Work out the finished part from the listing and answer in its coordinate system (mm). Face numbers are marked on the shaded views. Give positions to 0.01 mm unless a question says otherwise; leave off trailing zeros. Loops run counter-clockwise (first coordinate to the right, second up) from the corner with the lowest first, then second, coordinate; pieces in that order, holes last. Notation, with made-up numbers: (78, 76.5) - (132, 76.5) arc R23 ccw to (132, 94.5) - close; hole circle Ø6 at (89, -28.75). An arc over 180 degrees is marked (long way). One line per question, with ' | ' between items.
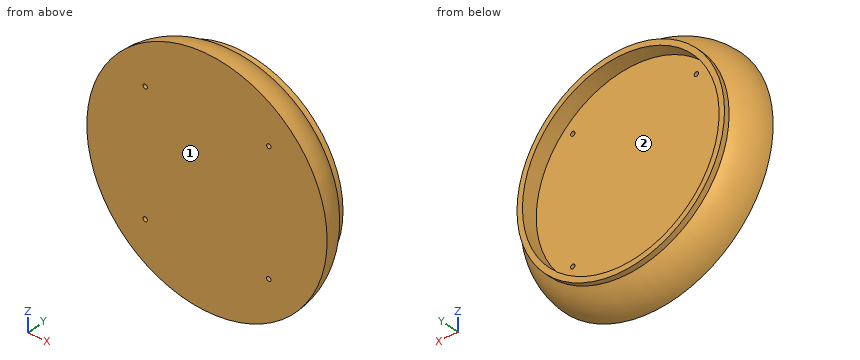
from build123d import *

# Parameters (mm, degrees)
SKETCH1_R          = 2
CUT_EXTRUDE1_DEPTH = 21


with BuildPart() as part:
    # Sketch2 → Revolve1 (revolve)
    with BuildSketch(Plane.XY):
        with BuildLine():
            Line((90, 0), (90, 15))
            Line((90, 15), (95, 15))
            Line((95, 15), (95, 10))
            ThreePointArc((95, 10), (106.041019662, -3.229490169), (110, -20))
            Line((110, -20), (0, -20))
            Line((0, -20), (0, 0))
            Line((0, 0), (90, 0))
        make_face()
    revolve(axis=Axis((0, 0, 0), (0, -1, 0)))

    # Sketch1 → Cut-Extrude1 (cut, through all)
    with BuildSketch(Plane(origin=(0, 0, 0), x_dir=(1, 0, 0), z_dir=(0, 1, 0))):
        with Locations((-56.568542495, 56.568542495)):
            Circle(SKETCH1_R)
        with Locations((-56.568542495, -56.568542495)):
            Circle(SKETCH1_R)
        with Locations((56.568542495, 56.568542495)):
            Circle(SKETCH1_R)
        with Locations((56.568542495, -56.568542495)):
            Circle(SKETCH1_R)
    extrude(amount=-CUT_EXTRUDE1_DEPTH, mode=Mode.SUBTRACT)


solid = part.part
1. Find section B-B on z = 0. Write down the section's boundary in (x, y), then the cut area to 3 significant figures.
Evaluation:
outline: (-110, -20) - (110, -20) arc R37.5 ccw to (95, 10) - (95, 15) - (90, 15) - (90, 0) - (-90, 0) - (-90, 15) - (-95, 15) - (-95, 10) arc R37.5 ccw to start | area: 4,580 mm2
2. Flat-ended cylindrical pins translate along their axes: pin 1 (4.5 mm diameter, centred on x = 56.57, z = 56.57, fed in from -Y); pin 2 (2 mm diameter, centred on y = -15.5, z = -26, fed in from -X); pin 3 (3 mm diameter, centred on x = 64, z = 37, fed in from +Y); pin 4 (4 mm diameter, centred on y = 10, z = -54.5, fed in from +X). Find the tip coordinate at first contact, or state that the pin passes through.
Evaluation:
pin 1: y = -20 | pin 2: x = -106.87 | pin 3: y = 0 | pin 4: x = 81.09
3. Find section C-C on y = -5. Write down the section's boundary in (x, z), then the cut area to 3 significant figures.
Evaluation:
outline: circle Ø213.74 at (0, 0); hole circle Ø4 at (-56.57, -56.57); hole circle Ø4 at (-56.57, 56.57); hole circle Ø4 at (56.57, -56.57); hole circle Ø4 at (56.57, 56.57) | area: 35,800 mm2
4. Consider L1, parallel to Z at x = -55, y = -5; L2, parallel to X at y = -15, z = -58; L3, parallel to Y at x = 10, z = 48.5. Determine where each line is inside the solid, lowest interval first.
Evaluation:
L1: -91.63 to -57.81, -55.33 to 55.33, 57.81 to 91.63 | L2: -93.07 to -57.97, -55.17 to 55.17, 57.97 to 93.07 | L3: -20 to 0
5. Find section A-A on x = 0. Write down the section's boundary in (y, z).
Evaluation:
outline: (-20, -110) arc R37.5 ccw to (10, -95) - (15, -95) - (15, -90) - (0, -90) - (0, 90) - (15, 90) - (15, 95) - (10, 95) arc R37.5 ccw to (-20, 110) - close
6. Determine the mould class of the marked faces 1 and 2 for opening direction Z: +Z half, -Z half, draft (parallel to the pull), parting line (faces both ways), or undercut.
Evaluation:
face 1: draft | face 2: undercut
